from build123d import *

# Parameters (mm, degrees)
SKETCH1_R           = 2.25
BOSS_EXTRUDE1_DEPTH = 5.5
SKETCH1_3_R         = 1.25
BOSS_EXTRUDE2_DEPTH = 1
SKETCH5_R           = 1.25
BOSS_EXTRUDE3_DEPTH = 1
SKETCH6_R           = 2
BOSS_EXTRUDE4_DEPTH = 1
SKETCH12_R          = 1.25
CUT_EXTRUDE1_DEPTH  = 5


with BuildPart() as part:
    # Sketch1 → Boss-Extrude1 (new body)
    with BuildSketch(Plane(origin=(0, 0, 0), x_dir=(1, 0, 0), z_dir=(0, 1, 0))):
        with Locations((-0.522013312, 0.511138034)):
            Circle(SKETCH1_R)
    extrude(amount=BOSS_EXTRUDE1_DEPTH)

    # Sketch1<3> → Boss-Extrude2 (add)
    with BuildSketch(Plane(origin=(0, 0, 0), x_dir=(1, 0, 0), z_dir=(0, 1, 0))):
        with Locations((-0.522013312, 0.511138034)):
            Circle(SKETCH1_3_R)
    extrude(amount=BOSS_EXTRUDE2_DEPTH)

    # Sketch5 → Boss-Extrude3 (add)
    with BuildSketch(Plane.XZ):
        with Locations((-0.522013312, -0.511138034)):
            Circle(SKETCH5_R)
    extrude(amount=BOSS_EXTRUDE3_DEPTH)

    # Sketch6 → Boss-Extrude4 (add)
    with BuildSketch(Plane.XZ.offset(1)):
        with Locations((-0.522013312, -0.511138034)):
            Circle(SKETCH6_R)
    extrude(amount=BOSS_EXTRUDE4_DEPTH)

    # Sketch12 → Cut-Extrude1 (cut)
    with BuildSketch(Plane(origin=(0, 5.5, 0), x_dir=(1, 0, 0), z_dir=(0, 1, 0))):
        with Locations((-0.522013312, 0.511138034)):
            Circle(SKETCH12_R)
    extrude(amount=-CUT_EXTRUDE1_DEPTH, mode=Mode.SUBTRACT)


solid = part.part
CAD build for the part. Positions are in the model's coordinates, mm. A direction names the side the tool comes from. Coordinates: 2 decimals unless noted, no trailing zeros. Write each loop counter-clockwise with the first axis right and the second up, starting at its lowest first coordinate (ties: lowest second). Pieces come first, ordered by that corner, then holes. Notation, with made-up numbers: M 9,-11 L 48,-11 A29 ccw 48,15 Z; hole C 36,54.25 d9. An arc over 180 degrees is marked long. Return JSON: item names as keys, results as strings.
Item 1: Probe line 1 (Y direction, x = 0.9, z = 0.6); line 2 (X direction, y = 3, z = 0.45); line 3 (Z direction, x = -1.45, y = 4). List the from-to ranges inside material, lowest first. Write a range as from..to.
Findings below:
{"line 1": "y = -2..-1, 0..5.5", "line 2": "x = -2.56..-1.32, 0.28..1.51", "line 3": "z = -2.56..-1.35, 0.33..1.54"}
Item 2: Which spindle directions (+Z, -Z, +X, -X, +Y, -Y) get a long thin tool onto all of the face, cutting with end or side? Do faces 5 (the cylindrical face through (-2.308, 2.712, 0.858)), 6 (the cylindrical face through (1.325, -1.493, -1.277)), 7 (the cylindrical face through (-1.514, -0.493, -1.272)), 8 (the flat face through (-1, -2, 0)), 9 (the flat face through (-1, 0.5, -1)). Say none if no direction does.
Findings below:
{"face 5": "+Y, -Y", "face 6": "-Y", "face 7": "none", "face 8": "+Z, -Z, +X, -X, -Y", "face 9": "+Y"}
Item 3: Slice it at C-C, the plane x = 0.45. Write the cut outline in (y, z).
Findings below:
{"outline": "M -2,-2.26 L -1,-2.26 L -1,-1.3 L 0,-1.3 L 0,-2.54 L 5.5,-2.54 L 5.5,-1.3 L 0.5,-1.3 L 0.5,0.27 L 5.5,0.27 L 5.5,1.52 L 0,1.52 L 0,0.27 L -1,0.27 L -1,1.24 L -2,1.24 Z"}
Item 4: Slice it at B-B, the plane x = 1.15. Write the cut outline in (y, z).
Findings below:
{"outline": "M -2,-1.61 L -1,-1.61 L -1,0.59 L -2,0.59 Z; M 0,-2.02 L 5.5,-2.02 L 5.5,0.99 L 0,0.99 Z"}
Item 5: Drop a flat-ended pin along its axis: pin 1 Ø2 at (x, z) = (-1, 0) entering from +Y. Give the stop position or say it passes through.
Findings below:
{"pin 1": "stops at y = 5.5"}
Item 6: Slice it at A-A, the plane z = 1.2. Write the cut outline in (x, y).
Findings below:
{"outline": "M -1.98,0 L 0.94,0 L 0.94,5.5 L -1.98,5.5 Z; M -1.56,-2 L 0.51,-2 L 0.51,-1 L -1.56,-1 Z"}
Item 7: Slice it at D-D, the plane z = -0.4. Write the cut outline in (x, y).
Findings below:
{"outline": "M -2.77,0 L -1.77,0 L -1.77,-1 L -2.52,-1 L -2.52,-2 L 1.47,-2 L 1.47,-1 L 0.72,-1 L 0.72,0 L 1.73,0 L 1.73,5.5 L 0.72,5.5 L 0.72,0.5 L -1.77,0.5 L -1.77,5.5 L -2.77,5.5 Z"}
Item 8: Two-plate mould, pull along Y, no slides. Class faces 1 (the flat face through (1, -1, 0)), 2 (the flat face through (-1, 5.5, 1)), 3 (the flat face through (-1, 0, 1)), 4 (the cylindrical face through (-1.4, 3, -1.4)): +Y half, -Y half, draft (parallel to the pull), parting line (faces both ways), or undercut.
Findings below:
{"face 1": "undercut", "face 2": "+Y half", "face 3": "undercut", "face 4": "draft"}
